Build history of the part. All positions in model axes, mm. Give positions to 0.01 mm unless a question says otherwise; leave off trailing zeros. Loops run counter-clockwise (first coordinate to the right, second up) from the corner with the lowest first, then second, coordinate; pieces in that order, holes last. Notation, with made-up numbers: (82, 21) -> (102, 21) arc R7 ccw to (102, 33) -> close; hole circle Ø6 at (-11.5, -21.5). An arc over 180 degrees is marked (long way). One line per question, with ' | ' between items. Start each with the question number.
(1) Slice it at D-D, the plane x = 180. Write the cut outline in (y, z), then the cut area to 3 significant figures.
(2) Slice it at B-B, the plane z = 28. Write the cut outline in (x, y), then the cut area to 3 significant figures.
(3) Drill centre lines: L1, parallel to X at y = -1.95, z = 97; L2, parallel to X at y = -2.4, z = 58.5; L3, parallel to Z at x = -143, y = -3.95. Where is each one in solid material? Low to high. Write a range as from..to.
(4) Slice it at A-A, the plane x = 98.5. Write the cut outline in (y, z), then the cut area to 3 significant figures.
(5) Slice it at C-C, the plane y = -4. Give the number of separate pieces and of enclosed holes in the cut face, then the cut area to 3 significant figures.
```python
from build123d import *

# Parameters (mm, degrees)
F0_W     = 600
F0_H     = 320
F0_R     = 95
F1_DEPTH = 5
F2_R     = 2.5
F3_DEPTH = 25
F4_R     = 4
F5_DEPTH = 25


with BuildPart() as f1:
    # F0 (on Front) → F1 (new body)
    with BuildSketch(Plane.XZ):
        Rectangle(F0_W, F0_H)
        with Locations((-119.303569, 45)):
            Circle(F0_R, mode=Mode.SUBTRACT)
        with Locations((120.696431, 45)):
            Circle(F0_R, mode=Mode.SUBTRACT)
    extrude(amount=F1_DEPTH)

    # F2 (on face) → F3 (cut)
    with BuildSketch(Plane.XZ.offset(5)):
        with Locations((-120.931181, 143.486552)):
            Circle(F2_R)
        with Locations((118.338796, 143.471781)):
            Circle(F2_R)
        with Locations((-190.094973, 113.489613)):
            Circle(F2_R)
        with Locations((-217.790121, 43.372388)):
            Circle(F2_R)
        with Locations((-187.793182, -25.791404)):
            Circle(F2_R)
        with Locations((-117.675957, -53.486552)):
            Circle(F2_R)
        with Locations((-48.512165, -23.489613)):
            Circle(F2_R)
        with Locations((-20.817017, 46.627612)):
            Circle(F2_R)
        with Locations((-50.813956, 115.791404)):
            Circle(F2_R)
        with Locations((49.399267, 112.962964)):
            Circle(F2_R)
        with Locations((22.22465, 42.642365)):
            Circle(F2_R)
        with Locations((52.733467, -26.297164)):
            Circle(F2_R)
        with Locations((123.054066, -53.471781)):
            Circle(F2_R)
        with Locations((191.993594, -22.962964)):
            Circle(F2_R)
        with Locations((219.168211, 47.357635)):
            Circle(F2_R)
        with Locations((188.659395, 116.297164)):
            Circle(F2_R)
    extrude(amount=-F3_DEPTH, mode=Mode.SUBTRACT)

    # F4 (on face) → F5 (cut)
    with BuildSketch(Plane(origin=(0, 0, 0), x_dir=(-1, 0, 0), z_dir=(0, 1, 0))):
        with Locations((289.000004, 149.000004)):
            Circle(F4_R)
        with Locations((289.000004, -148.999996)):
            Circle(F4_R)
        with Locations((144.500004, 149.000004)):
            Circle(F4_R)
        with Locations((144.500004, -148.999996)):
            Circle(F4_R)
        with Locations((4e-06, 149.000004)):
            Circle(F4_R)
        with Locations((4e-06, -148.999996)):
            Circle(F4_R)
        with Locations((-144.499996, 149.000004)):
            Circle(F4_R)
        with Locations((-144.499996, -148.999996)):
            Circle(F4_R)
        with Locations((-288.999996, 149.000004)):
            Circle(F4_R)
        with Locations((-288.999996, -148.999996)):
            Circle(F4_R)
        with Locations((-289.000004, 0)):
            Circle(F4_R)
        with Locations((289.000004, 4e-06)):
            Circle(F4_R)
    extrude(amount=-F5_DEPTH, mode=Mode.SUBTRACT)


solid = f1.part
```
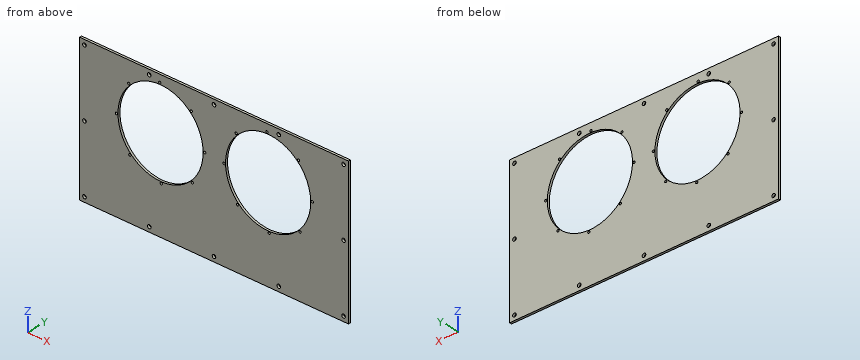
Final values:
1) outline: (-5, -160) -> (0, -160) -> (0, -29.22) -> (-5, -29.22) -> close; (-5, 119.22) -> (0, 119.22) -> (0, 160) -> (-5, 160) -> close | area: 858 mm2
2) outline: (-300, -5) -> (-212.77, -5) -> (-212.77, 0) -> (-300, 0) -> close; (-25.84, -5) -> (27.23, -5) -> (27.23, 0) -> (-25.84, 0) -> close; (214.16, -5) -> (300, -5) -> (300, 0) -> (214.16, 0) -> close | area: 1,130 mm2
3) L1: -300..-198.81, -39.8..41.19, 200.2..300 | L2: -300..-213.34, -25.27..26.66, 214.73..300 | L3: -160..-152.71, -145.29..-47, 137..145.29, 152.71..160
4) outline: (-5, -160) -> (0, -160) -> (0, -47.37) -> (-5, -47.37) -> close; (-5, 137.37) -> (0, 137.37) -> (0, 160) -> (-5, 160) -> close | area: 676 mm2
5) separate pieces: 1 | enclosed holes: 30 | area: 134,000 mm2
